Part model, mm, in its own coordinate system. Face numbers are marked on the shaded views. A direction names the side the tool comes from. Give positions to 0.01 mm unless a question says otherwise; leave off trailing zeros. Write each loop counter-clockwise with the first axis right and the second up, starting at its lowest first coordinate (ties: lowest second). Pieces come first, ordered by that corner, then holes. Notation, with made-up numbers: M -33.5,30 L 4.5,30 A8 cw 4.5,43 Z; hole C 30.5,25 d8. An arc over 180 degrees is marked long. Use CSV: the item, a comma, the result in double quotes. Start each with the question number.
Item 1: Mould opens along Y. For the marked faces 1, 2, 3 and 4 say: released by +Y, released by -Y, zero draft, split by the parting line, or undercut.
Item 2: Pin check, flat tips, straight feed: pin 1 (0.8 mm diameter, centred on y = -36.5, z = 9, fed in from +X); pin 2 (3 mm diameter, centred on y = -36.5, z = 7, fed in from -X); pin 3 (10 mm diameter, centred on x = 14, y = -14, fed in from +Z). Stop position of each tip, or through.
Item 3: Cut at D-D (x = 16.5). List the corners of the cut face in (y, z) (3 decimals), then the cut area to 3 significant figures.
Item 4: Cut at A-A (z = 9.5). List the corners of the cut face in (x, y) (3 decimals), then the cut area to 3 significant figures.
Item 5: Drill centre lines: line 1 (Y direction, x = 0, z = 0.05) (3 decimals); line 2 (Z direction, x = -24, y = -28); line 3 (X direction, y = 30, z = 0.05). Where is each one in solid material? Low to high. Write a range as [from, to].
Item 6: Cut at C-C (x = 0). Count the separate pieces of the cut face and the enclosed holes in it, then the cut area to 3 significant figures.
Item 7: Which spindle directions (+Z, -Z, +X, -X, +Y, -Y) get a long thin tool onto all of the face, cutting with end or side? Do the marked faces 5 and 6. Say none if no direction does.
from build123d import *

# Parameters (mm, degrees)
SKETCH_1_W          = 56
SKETCH_1_H          = 75.65
EXTRUDE_1_DEPTH     = 2
SKETCH_2_W          = 5
SKETCH_2_H          = 1.8
EXTRUDE_2_DEPTH     = 19.3
EXTRUDE_3_DEPTH     = 5
EXTRUDE_4_DEPTH     = 5
EXTRUDE_5_DEPTH     = 5
EXTRUDE_6_DEPTH     = 5
SKETCH_7_R          = 1.6
CUT_EXTRUDE_1_DEPTH = 51.864728693
CHAMFER_1_SIZE      = 2


with BuildPart() as part:
    # 草图1 → 凸台-拉伸1 (new body)
    with BuildSketch(Plane.XY):
        Rectangle(SKETCH_1_W, SKETCH_1_H)
    extrude(amount=EXTRUDE_1_DEPTH)

    # 草图2 → 凸台-拉伸2 (add)
    with BuildSketch(Plane.XY.offset(2)):
        with Locations((-25, 36.925)):
            Rectangle(SKETCH_2_W, SKETCH_2_H)
        with Locations((25, 36.925)):
            Rectangle(SKETCH_2_W, SKETCH_2_H)
        with Locations((-25, -36.925)):
            Rectangle(SKETCH_2_W, SKETCH_2_H)
        with Locations((25, -36.925)):
            Rectangle(SKETCH_2_W, SKETCH_2_H)
    extrude(amount=EXTRUDE_2_DEPTH)

    # 草图3 → 凸台-拉伸3 (add)
    with BuildSketch(Plane.ZY.offset(27.5)):
        Polygon((21.3, 36.025), (19.3, 35.025), (19.3, 36.025), align=None)
    extrude(amount=-EXTRUDE_3_DEPTH)

    # 草图4 → 凸台-拉伸4 (add)
    with BuildSketch(Plane.ZY.offset(-22.5)):
        Polygon((19.3, 36.025), (19.3, 35.025), (21.3, 36.025), align=None)
    extrude(amount=-EXTRUDE_4_DEPTH)

    # 草图5 → 凸台-拉伸5 (add)
    with BuildSketch(Plane.ZY.offset(27.5)):
        Polygon((21.3, -36.025), (19.3, -35.025), (19.3, -36.025), align=None)
    extrude(amount=-EXTRUDE_5_DEPTH)

    # 草图6 → 凸台-拉伸6 (add)
    with BuildSketch(Plane.ZY.offset(-22.5)):
        Polygon((19.3, -36.025), (21.3, -36.025), (19.3, -35.025), align=None)
    extrude(amount=-EXTRUDE_6_DEPTH)

    # 草图7 → 切除-拉伸1 (cut, through all)
    with BuildSketch(Plane.XY.offset(2)):
        with Locations((0, 30)):
            Circle(SKETCH_7_R)
        with Locations((0, -30)):
            Circle(SKETCH_7_R)
    extrude(amount=-CUT_EXTRUDE_1_DEPTH, mode=Mode.SUBTRACT)

    # 倒角1
    chamfer_1_edges = [part.edges().sort_by_distance(p)[0] for p in [
        (-1.6, 30, 2),
        (-1.6, -30, 2),
    ]]
    chamfer(chamfer_1_edges, length=CHAMFER_1_SIZE - 0.0001)  # a hair under: the kernel refuses the full size


solid = part.part
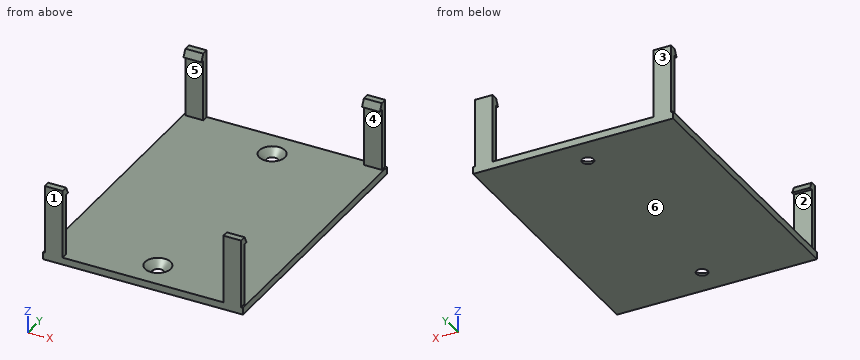
Worked answers:
1,face 1,"released by -Y"
1,face 2,"undercut"
1,face 3,"released by +Y"
1,face 4,"undercut"
2,pin 1,"stops at x = 27.5"
2,pin 2,"stops at x = -27.5"
2,pin 3,"stops at z = 2"
3,outline,"M -37.825,0 L 37.825,0 L 37.825,2 L -37.825,2 Z"
3,area,"151 mm^2"
4,outline,"M -27.5,-37.825 L -22.5,-37.825 L -22.5,-36.025 L -27.5,-36.025 Z; M -27.5,36.025 L -22.5,36.025 L -22.5,37.825 L -27.5,37.825 Z; M 22.5,-37.825 L 27.5,-37.825 L 27.5,-36.025 L 22.5,-36.025 Z; M 22.5,36.025 L 27.5,36.025 L 27.5,37.825 L 22.5,37.825 Z"
4,area,"36.0 mm^2"
5,line 1,"y = [-37.825, -31.65], [-28.35, 28.35], [31.65, 37.825]"
5,line 2,"z = [0, 2]"
5,line 3,"x = [-28, -1.65], [1.65, 28]"
6,separate pieces,"3"
6,enclosed holes,"0"
6,area,"131 mm^2"
7,face 5,"+X, -X"
7,face 6,"-Z, +X, -X, +Y, -Y"
